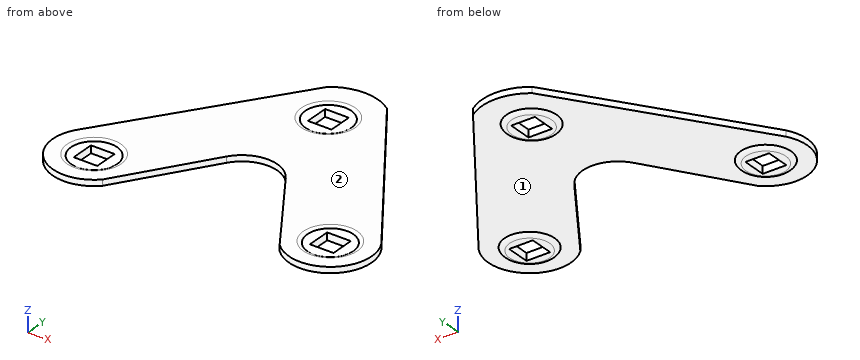
from build123d import *

# Parameters (mm, degrees)
BOSS_EXTRUDE2_DEPTH = 1
SKETCH2_R           = 3.9
CUT_EXTRUDE1_DEPTH  = 0.25
FILLET1_R           = 1
SKETCH5_W           = 4
SKETCH5_H           = 4
CUT_EXTRUDE6_DEPTH  = 2
SKETCH6_R           = 4.25
SKETCH6_W           = 4
SKETCH6_H           = 4
BOSS_EXTRUDE3_DEPTH = 0.5
FILLET2_R           = 1


with BuildPart() as part:
    # Sketch1 → Boss-Extrude2 (new body)
    with BuildSketch(Plane.XY):
        with BuildLine():
            Line((-5, 12.31662479), (-15, -2.758942439))
            ThreePointArc((-15, -2.758942439), (-24.276770595, -3.401554175), (-26.006226146, 5.735207068))
            Line((-26.006226146, 5.735207068), (-5, 35.735207068))
            ThreePointArc((-5, 35.735207068), (0, 37.388266463), (5, 35.735207068))
            Line((5, 35.735207068), (26.006226146, 5.735207068))
            ThreePointArc((26.006226146, 5.735207068), (24.276770595, -3.401554175), (15, -2.758942439))
            Line((15, -2.758942439), (5, 12.31662479))
            ThreePointArc((5, 12.31662479), (0, 15), (-5, 12.31662479))
        make_face()
    extrude(amount=BOSS_EXTRUDE2_DEPTH)

    # Sketch2 → Cut-Extrude1 (cut)
    with BuildSketch(Plane.XY.offset(1)):
        with Locations((-20, 2.140037047)):
            Circle(SKETCH2_R)
        with Locations((20, 2.140037047)):
            Circle(SKETCH2_R)
        with Locations((0, 29)):
            Circle(SKETCH2_R)
    extrude(amount=-CUT_EXTRUDE1_DEPTH, mode=Mode.SUBTRACT)

    # Fillet1
    # the kernel refuses this fillet: 1 mm, written as the material it takes off along each edge
    with BuildSketch(Plane(origin=(-20, 2.140037047, 1), x_dir=(1, 0, 0), z_dir=(0, -1, 0))) as fillet1_piece_1:
        with BuildLine():
            CenterArc((4.561437828, -1), FILLET1_R, 90, 41.409622109)
            Line((3.9, -0.25), (3.886771243, -0.235))
            ThreePointArc((3.886771243, -0.235), (3.88, -0.125), (3.88, 0))
            Line((3.88, 0), (3.9, 0.02))
            Line((3.9, 0.02), (4.561437828, 0.02))
            Line((4.561437828, 0.02), (4.561437828, 0))
        make_face()
    revolve(axis=Axis((-20, 2.140037047, 1), (0, 0, 1)), mode=Mode.SUBTRACT)
    with BuildSketch(Plane(origin=(20, 2.140037047, 1), x_dir=(1, 0, 0), z_dir=(0, -1, 0))) as fillet1_piece_2:
        with BuildLine():
            CenterArc((4.561437828, -1), FILLET1_R, 90, 41.409622109)
            Line((3.9, -0.25), (3.886771243, -0.235))
            ThreePointArc((3.886771243, -0.235), (3.88, -0.125), (3.88, 0))
            Line((3.88, 0), (3.9, 0.02))
            Line((3.9, 0.02), (4.561437828, 0.02))
            Line((4.561437828, 0.02), (4.561437828, 0))
        make_face()
    revolve(axis=Axis((20, 2.140037047, 1), (0, 0, 1)), mode=Mode.SUBTRACT)
    with BuildSketch(Plane(origin=(0, 29, 1), x_dir=(1, 0, 0), z_dir=(0, -1, 0))) as fillet1_piece_3:
        with BuildLine():
            CenterArc((4.561437828, -1), FILLET1_R, 90, 41.409622109)
            Line((3.9, -0.25), (3.886771243, -0.235))
            ThreePointArc((3.886771243, -0.235), (3.88, -0.125), (3.88, 0))
            Line((3.88, 0), (3.9, 0.02))
            Line((3.9, 0.02), (4.561437828, 0.02))
            Line((4.561437828, 0.02), (4.561437828, 0))
        make_face()
    revolve(axis=Axis((0, 29, 1), (0, 0, 1)), mode=Mode.SUBTRACT)

    # Sketch5 → Cut-Extrude6 (cut)
    with BuildSketch(Plane.XY.offset(1)):
        with Locations((0, 29)):
            Rectangle(SKETCH5_W, SKETCH5_H)
        with Locations((20, 2.140037047)):
            Rectangle(SKETCH5_W, SKETCH5_H)
        with Locations((-20, 2.140037047)):
            Rectangle(SKETCH5_W, SKETCH5_H)
    extrude(amount=-CUT_EXTRUDE6_DEPTH, mode=Mode.SUBTRACT)

    # Sketch6 → Boss-Extrude3 (add)
    # profile 1 of 3: a face of its own
    with BuildSketch(Plane(origin=(0, 0, 0), x_dir=(-1, 0, 0), z_dir=(0, 0, -1))):
        with Locations((0, 29)):
            Circle(SKETCH6_R)
        with Locations((0, 29)):
            Rectangle(SKETCH6_W, SKETCH6_H, mode=Mode.SUBTRACT)
    # profile 2 of 3: a face of its own
    with BuildSketch(Plane(origin=(0, 0, 0), x_dir=(-1, 0, 0), z_dir=(0, 0, -1))):
        with Locations((-20, 2.140037047)):
            Circle(SKETCH6_R)
        with Locations((-20, 2.140037047)):
            Rectangle(SKETCH6_W, SKETCH6_H, mode=Mode.SUBTRACT)
    # profile 3 of 3: a face of its own
    with BuildSketch(Plane(origin=(0, 0, 0), x_dir=(-1, 0, 0), z_dir=(0, 0, -1))):
        with Locations((20, 2.140037047)):
            Circle(SKETCH6_R)
        with Locations((20, 2.140037047)):
            Rectangle(SKETCH6_W, SKETCH6_H, mode=Mode.SUBTRACT)
    extrude(amount=BOSS_EXTRUDE3_DEPTH)

    # Fillet2
    # the kernel refuses this fillet: 1 mm, written as the material it takes off along each edge
    with BuildSketch(Plane(origin=(0, 29, -0.5), x_dir=(-1, 0, 0), z_dir=(0, -1, 0))) as fillet2_piece_1:
        with BuildLine():
            CenterArc((3.383974596, -1), FILLET2_R, 30, 60)
            Line((4.25, -0.5), (4.267320508, -0.49))
            ThreePointArc((4.267320508, -0.49), (4.27, -0.25), (4.27, 0))
            Line((4.27, 0), (4.25, 0.02))
            Line((4.25, 0.02), (3.383974596, 0.02))
            Line((3.383974596, 0.02), (3.383974596, 0))
        make_face()
    revolve(axis=Axis((0, 29, -0.5), (0, 0, -1)), mode=Mode.SUBTRACT)
    with BuildSketch(Plane(origin=(20, 2.140037047, -0.5), x_dir=(-1, 0, 0), z_dir=(0, -1, 0))) as fillet2_piece_2:
        with BuildLine():
            CenterArc((3.383974596, -1), FILLET2_R, 30, 60)
            Line((4.25, -0.5), (4.267320508, -0.49))
            ThreePointArc((4.267320508, -0.49), (4.27, -0.25), (4.27, 0))
            Line((4.27, 0), (4.25, 0.02))
            Line((4.25, 0.02), (3.383974596, 0.02))
            Line((3.383974596, 0.02), (3.383974596, 0))
        make_face()
    revolve(axis=Axis((20, 2.140037047, -0.5), (0, 0, -1)), mode=Mode.SUBTRACT)
    with BuildSketch(Plane(origin=(-20, 2.140037047, -0.5), x_dir=(-1, 0, 0), z_dir=(0, -1, 0))) as fillet2_piece_3:
        with BuildLine():
            CenterArc((3.383974596, -1), FILLET2_R, 30, 60)
            Line((4.25, -0.5), (4.267320508, -0.49))
            ThreePointArc((4.267320508, -0.49), (4.27, -0.25), (4.27, 0))
            Line((4.27, 0), (4.25, 0.02))
            Line((4.25, 0.02), (3.383974596, 0.02))
            Line((3.383974596, 0.02), (3.383974596, 0))
        make_face()
    revolve(axis=Axis((-20, 2.140037047, -0.5), (0, 0, -1)), mode=Mode.SUBTRACT)


solid = part.part
Model file for the job. Use its own axes, mm. Face numbers are marked on the shaded views. Give positions to 0.01 mm unless a question says otherwise; leave off trailing zeros. Loops run counter-clockwise (first coordinate to the right, second up) from the corner with the lowest first, then second, coordinate; pieces in that order, holes last.
1) Saw through at A-A (z = 0.3). Write the cut outline in (x, y).
2) Saw through at B-B (x = 20). Write the cut outline in (y, z), plus the area to 3 significant figures.
3) Wall check: line 1 (Z direction, x = -11, y = 10.5); line 2 (X direction, y = -2.5, z = 0.6); line 3 (X direction, y = 10.5, z = 0.8). Give the ranges that are in metal, low to high.
4) Pull direction Z, two halves, no side cores. Call the marked faces 1 and 2: +Z half, -Z half, draft (parallel to the pull), parting line (faces both ways), or undercut.
5) Flat gauge pins, fed straight in: pin 1 Ø0.6 at (x, z) = (20.5, 0) entering from -Y; pin 2 Ø0.6 at (x, z) = (-20.5, 0) entering from +Y; pin 3 Ø0.6 at (y, z) = (29, 0.5) entering from +X. Where does each tip first touch, or does it go through?
6) Saw through at C-C (y = 11.5). Write the cut outline in (x, z), plus the area to 3 significant figures.
7) Saw through at D-D (x = 7.5). Write the cut outline in (y, z).
Answer block:
1. outline: (-26.01, 5.74) arc R7 ccw to (-15, -2.76) - (-5, 12.32) arc R6 cw to (5, 12.32) - (15, -2.76) arc R7 ccw to (26.01, 5.74) - (5, 35.74) arc R8.39 ccw to (-5, 35.74) - close; hole (-22, 0.14) - (-18, 0.14) - (-18, 4.14) - (-22, 4.14) - close; hole (-2, 27) - (2, 27) - (2, 31) - (-2, 31) - close; hole (18, 0.14) - (22, 0.14) - (22, 4.14) - (18, 4.14) - close
2. outline: (-4.86, 0) - (-2.11, 0) arc R1 ccw to (-1.24, -0.5) - (0.14, -0.5) - (0.14, 0.75) - (-1.76, 0.75) arc R1 ccw to (-2.42, 1) - (-4.86, 1) - close; (4.14, -0.5) - (5.52, -0.5) arc R1 ccw to (6.39, 0) - (14.31, 0) - (14.31, 1) - (6.7, 1) arc R1 ccw to (6.04, 0.75) - (4.14, 0.75) - close
2. area: 16.1 mm2
3. line 1: z = 0 to 1
3. line 2: x = -25.24 to -14.83, 14.83 to 25.24
3. line 3: x = -22.67 to -6.21, 6.21 to 22.67
4. face 1: -Z half
4. face 2: +Z half
5. pin 1: stops at y = -4.86
5. pin 2: stops at y = 14.03
5. pin 3: stops at x = 9.93
6. outline: (-21.97, 0) - (-5.54, 0) - (-5.54, 1) - (-21.97, 1) - close; (5.54, 0) - (21.97, 0) - (21.97, 1) - (5.54, 1) - close
6. area: 32.9 mm2
7. outline: (8.55, 0) - (32.16, 0) - (32.16, 1) - (8.55, 1) - close
